Part model, mm, in its own coordinate system. A direction names the side the tool comes from. Round coordinates to 2 decimals unless told otherwise and drop trailing zeros. Order: outer loops, then holes, each group sorted by start corner. A loop starts at its lowest first (then second) coordinate and runs counter-clockwise, first axis right, second up. Notation, with made-up numbers: (79, -14.75) - (123, -14.75) arc R17 ccw to (123, 4.25) - close; hole circle Ø4 at (68, 3.5). An arc over 180 degrees is marked (long way). Return JSON: item names as keys, results as strings. Group by question number.
Item 1: Saw through at D-D on y = -6. List the corners of the cut face in (x, z).
Item 2: Saw through at C-C on z = -1. List the corners of the cut face in (x, y), and give its area (3 significant figures).
Item 3: Saw through at B-B on z = -19. List the corners of the cut face in (x, y), and give its area (3 significant figures).
Item 4: Drop flat-ended pins along their axis: pin 1 (8 mm diameter, centred on y = 0, z = -19, fed in from +X); pin 2 (4 mm diameter, centred on x = -0.5, y = 1.5, fed in from +Z); pin 3 (5.5 mm diameter, centred on y = 0, z = -19, fed in from +X); pin 4 (4 mm diameter, centred on x = 37, y = -1.5, fed in from -Z). Give the stop position or say it passes through.
Item 5: Probe probe 1 along X at (y, z) = (-1.25, -1); probe 2 along X at (y, z) = (4.25, -22); probe 3 along Y at (x, z) = (-36, 10). List the from-to ranges inside material, lowest first.
Item 6: Tool access for faces 4 (the face through (36, 0, -13)), 5 (the face through (-36, 0, -13)), 6 (the face through (15, 0, 7)), 7 (the face through (-14.5, 0, -15)): list every direction of +Z, -Z, +X, -X, +Y, -Y with a clear straight run to the whole face (end or side of a thin tool).
Item 7: Two-plate mould, pull along X, no slides. Class faces 1 (the face through (29.5, 2, -22)), 2 (the face through (-29.5, 2, -16)), 3 (the face through (-21.077, -0.112, -2.172)): released by +X, released by -X, zero draft, split by the parting line, or undercut.
Item 8: Saw through at A-A on z = -14.5. List the corners of the cut face in (x, y), and give its area (3 significant figures).
```python
from build123d import *

# Parameters (mm, degrees)
SKETCH_1_R             = 9
EXTRUDE_1_DEPTH        = 8
SKETCH_7_R             = 3.05
CUT_EXTRUDE_1_DEPTH    = 77.165937269
CUT_EXTRUDE_2_REACH    = 53.43
SKETCH_10_W            = 30
SKETCH_10_H            = 12
HOLE_WIZARD_M3_1_D     = 2.5
HOLE_WIZARD_M3_1_DEPTH = 8.5
HOLE_WIZARD_M3_1_TIP   = 0.751075774


with BuildPart() as part:
    # 草图1 → 凸台-拉伸1 (new, symmetric)
    with BuildSketch(Plane(origin=(0, 0, 0), x_dir=(1, 0, 0), z_dir=(0, 1, 0))):
        Polygon((-42, -13), (42, -13), (42, 13), (29.5, 13), (29.5, 25), (14.5, 25), (14.5, 9), (-14.5, 9), (-14.5, 25), (-29.5, 25), (-29.5, 13), (-42, 13), align=None)
        with Locations(Location((-30, 1, 0), (0, 0, 270))):
            Circle(SKETCH_1_R, mode=Mode.SUBTRACT)
        with Locations(Location((30, 1, 0), (0, 0, 90))):
            Circle(SKETCH_1_R, mode=Mode.SUBTRACT)
    extrude(amount=EXTRUDE_1_DEPTH, both=True)

    # 草图7 → 切除-拉伸1 (cut, through all)
    with BuildSketch(Plane.ZY.offset(29.5)):
        with Locations((-19, 0)):
            Circle(SKETCH_7_R)
    extrude(amount=-CUT_EXTRUDE_1_DEPTH, mode=Mode.SUBTRACT)

    # 草图10 → 切除-拉伸2 (cut, up to next)
    with BuildSketch(Plane.XZ.offset(8), mode=Mode.PRIVATE) as cut_extrude_2_sk1:
        with Locations((0, 7)):
            Rectangle(SKETCH_10_W, SKETCH_10_H)
    cut_extrude_2_tool1 = extrude(cut_extrude_2_sk1.sketch, amount=-CUT_EXTRUDE_2_REACH, mode=Mode.PRIVATE) & part.part
    add(cut_extrude_2_tool1.solids().sort_by_distance((0, -8, 7))[0], mode=Mode.SUBTRACT)

    # 草图8 → M4 螺纹孔1 (revolve, cut)
    with BuildSketch(Plane(origin=(42, 0, 10), x_dir=(0, 0, -1), z_dir=(0, 1, 0))):
        Polygon((0, 0), (0, 10.491420021), (1.65, 9.5), (1.65, 0), align=None)
    hole_wizard_m4_1 = revolve(axis=Axis((48.35, 0, 10), (-1, 0, 0)), mode=Mode.SUBTRACT)

    # 镜向1: M4 螺纹孔1 across plane
    add(hole_wizard_m4_1.mirror(Plane(origin=(0, 0, 0), x_dir=(0, 0, 1), z_dir=(1, 0, 0))), mode=Mode.SUBTRACT)

    # M3 螺纹孔1
    with Locations(Plane(origin=(0, 8, 0), x_dir=(1, 0, 0), z_dir=(0, 1, 0))):
        with Locations((-18.456603619, -6), (18.456603619, -6)):
            Hole(HOLE_WIZARD_M3_1_D / 2, depth=HOLE_WIZARD_M3_1_DEPTH)
            with Locations((0, 0, -(HOLE_WIZARD_M3_1_DEPTH + HOLE_WIZARD_M3_1_TIP / 2))):  # 118° drill point
                Cone(0, HOLE_WIZARD_M3_1_D / 2, HOLE_WIZARD_M3_1_TIP, mode=Mode.SUBTRACT)


solid = part.part
```
Filled in:
{
 "1": {"outline": "(-42, -13) - (-29.5, -13) - (-29.5, -25) - (-14.5, -25) - (-14.5, -9) - (14.5, -9) - (14.5, -25) - (29.5, -25) - (29.5, -13) - (42, -13) - (42, 13) - (15, 13) - (15, 1) - (-15, 1) - (-15, 13) - (-42, 13) - close; hole circle Ø18 at (-30, -1); hole circle Ø18 at (30, -1)"},
 "2": {"outline": "(-42, -8) - (-39, -8) - (-39, 8) - (-42, 8) - close; (-21, -8) - (21, -8) - (21, 8) - (-21, 8) - close; (39, -8) - (42, -8) - (42, 8) - (39, 8) - close", "area": "768 mm^2"},
 "3": {"outline": "(-29.5, -8) - (-14.5, -8) - (-14.5, -3.05) - (-29.5, -3.05) - close; (-29.5, 3.05) - (-14.5, 3.05) - (-14.5, 8) - (-29.5, 8) - close; (14.5, -8) - (29.5, -8) - (29.5, -3.05) - (14.5, -3.05) - close; (14.5, 3.05) - (29.5, 3.05) - (29.5, 8) - (14.5, 8) - close", "area": "297 mm^2"},
 "4": {"pin 1": "stops at x = 29.5", "pin 2": "stops at z = 1", "pin 3": "passes through", "pin 4": "stops at z = -13"},
 "5": {"probe 1": "x = -42 to -39, -21 to 21, 39 to 42", "probe 2": "x = -29.5 to -14.5, 14.5 to 29.5", "probe 3": "y = -8 to -1.65, 1.65 to 8"},
 "6": {"face 4": "-Z, +X, +Y, -Y", "face 5": "-Z, -X, +Y, -Y", "face 6": "+Z, +Y, -Y", "face 7": "-Z, +Y, -Y"},
 "7": {"face 1": "released by +X", "face 2": "released by -X", "face 3": "undercut"},
 "8": {"outline": "(-29.5, -8) - (-14.5, -8) - (-14.5, 8) - (-29.5, 8) - close; (14.5, -8) - (29.5, -8) - (29.5, 8) - (14.5, 8) - close", "area": "480 mm^2"}
}
